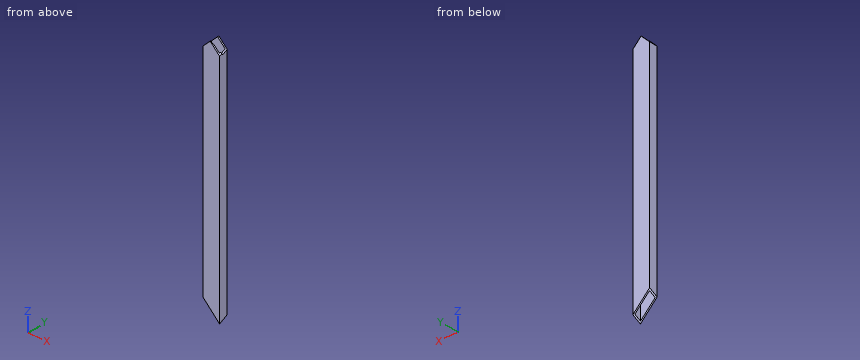
```python
from build123d import *

# Parameters (mm, degrees)
SKETCH1_W           = 50.8
SKETCH1_H           = 25.4
SKETCH1_W_2         = 44.45
SKETCH1_H_2         = 19.05
BOSS_EXTRUDE1_DEPTH = 771.9314
CUT_EXTRUDE1_DEPTH  = 773.76672179
CUT_EXTRUDE4_DEPTH  = 754.3292
CUT_EXTRUDE5_DEPTH  = 4.0132
SKETCH9_W           = 50.8
SKETCH9_H           = 21.0312
CUT_EXTRUDE7_DEPTH  = 16.8656
SKETCH10_W          = 77.733567683
SKETCH10_H          = 129.906903396
CUT_EXTRUDE8_DEPTH  = 40.64


with BuildPart() as part:
    # Sketch1 → Boss-Extrude1 (new body)
    with BuildSketch(Plane.XY):
        Rectangle(SKETCH1_W, SKETCH1_H)
        Rectangle(SKETCH1_W_2, SKETCH1_H_2, mode=Mode.SUBTRACT)
    extrude(amount=BOSS_EXTRUDE1_DEPTH)

    # Sketch2 → Cut-Extrude1 (cut, through all)
    with BuildSketch(Plane(origin=(0, 12.7, 0), x_dir=(1, 0, 0), z_dir=(0, 1, 0))):
        Polygon((25.4, 0), (-25.4, -50.8), (-25.4, 0), align=None)
        Polygon((-25.4, -771.9314), (25.4, -721.1314), (25.4, -771.9314), align=None)
    extrude(amount=-CUT_EXTRUDE1_DEPTH, mode=Mode.SUBTRACT)

    # Sketch5 → Cut-Extrude4 (cut)
    with BuildSketch(Plane(origin=(12.7, 0, -12.7), x_dir=(0, 1, 0), z_dir=(-0.7071067811865409, 0, 0.7071067811865541))):
        Polygon((12.7, -17.960512242), (12.7, -27.205356192), (-12.7, -17.960512242), align=None)
        Polygon((12.7, -527.877415309), (-12.7, -518.632571358), (-12.7, -527.877415309), align=None)
    extrude(amount=CUT_EXTRUDE4_DEPTH, mode=Mode.SUBTRACT)

    # Sketch7 → Cut-Extrude5 (cut)
    with BuildSketch(Plane(origin=(326.715708963, -168.170913211, 326.715708963), x_dir=(0.5736482337991444, -0.3364323186524704, -0.7468205934662252), z_dir=(0.6644630243886818, -0.3420201433256654, 0.6644630243886694))):
        Polygon((-595.337621849, -22.133397874), (-492.868446349, 40.706054593), (-475.594227989, 12.537844285), (-578.063403489, -50.301608182), align=None)
    extrude(amount=-CUT_EXTRUDE5_DEPTH, mode=Mode.SUBTRACT)

    # Sketch9 → Cut-Extrude7 (cut, symmetric)
    with BuildSketch(Plane(origin=(0, 0, 0), x_dir=(1, 0, 0), z_dir=(0, 1, 0))):
        with Locations((0, -755.37603578)):
            Rectangle(SKETCH9_W, SKETCH9_H)
    extrude(amount=CUT_EXTRUDE7_DEPTH, both=True, mode=Mode.SUBTRACT)

    # Sketch10 → Cut-Extrude8 (cut)
    with BuildSketch(Plane(origin=(-369.87845504, 0, 369.87845504), x_dir=(-0.7071067811865528, 0, -0.7071067811865422), z_dir=(0.7071067811865422, 0, -0.7071067811865528))):
        with Locations((-488.130578971, 23.675993241)):
            Rectangle(SKETCH10_W, SKETCH10_H)
    extrude(amount=-CUT_EXTRUDE8_DEPTH, mode=Mode.SUBTRACT)


solid = part.part
```
The listing builds one solid part. Answer for the finished solid, in the listing's coordinates (mm). Round coordinates to 2 decimals unless told otherwise and drop trailing zeros. Loops run counter-clockwise (first coordinate to the right, second up) from the corner with the lowest first, then second, coordinate; pieces in that order, holes last. Notation, with made-up numbers: (-28, 4) - (8, 4) arc R20 cw to (8, 28) - close; hole circle Ø4 at (-35.5, 23.25). An arc over 180 degrees is marked (long way). Return JSON: item names as keys, results as strings. Group by question number.
1. This flat-tipped pin is pushed along its axis until it touches: P1, Ø4, axis at x = 11, y = -6.5, coming from the -Z side (1 decimal). Where does it stop, or does it pass through?
2. The part is cut by section A-A on y = 4.25. Determine the outline of the cut face in (x, z) (3 decimals), then the cut area to 3 significant figures.
3. The part is cut by section C-C on x = 13. Determine the outline of the cut face in (y, z) (3 decimals), then the cut area to 3 significant figures.
4. The part is cut by section B-B on z = 112. Determine the outline of the cut face in (x, y) (3 decimals), then the cut area to 3 significant figures.
5. Consider probe 1 along X at (y, z) = (1.5, 182) (3 decimals); probe 2 along Y at (x, z) = (-14, 602) (3 decimals); probe 3 along Z at (x, y) = (-23, -4.75). Determine where each line is inside the solid, lowest interval first.
Resolved:
{
 "1": {"P1": "passes through"},
 "2": {"outline": "(-25.4, 59.525) - (-22.225, 56.35) - (-22.225, 717.532) - (-25.4, 714.357) - close; (22.225, 11.9) - (25.4, 8.725) - (25.4, 710.742) - (22.225, 713.917) - close", "area": "4,320 mm²"},
 "3": {"outline": "(-12.7, 12.4) - (-9.525, 14.034) - (-9.525, 722.091) - (-12.7, 720.457) - close; (9.525, 23.84) - (12.7, 25.474) - (12.7, 727.492) - (9.525, 725.857) - close", "area": "4,480 mm²"},
 "4": {"outline": "(-25.4, -12.7) - (25.4, -12.7) - (25.4, 12.7) - (-25.4, 12.7) - close; hole (-22.225, -9.525) - (22.225, -9.525) - (22.225, 9.525) - (-22.225, 9.525) - close", "area": "444 mm²"},
 "5": {"probe 1": "x = -25.4 to -22.225, 22.225 to 25.4", "probe 2": "y = -12.7 to -9.525, 9.525 to 12.7", "probe 3": "z = 52.49 to 716.76"}
}
